from build123d import *

# Parameters (mm, degrees)
F0_W     = 180
F0_H     = 50
F1_DEPTH = 2.5
F3_DEPTH = 60
F5_DEPTH = 50
F6_W     = 7.071068
F6_H     = 5
F7_DEPTH = 25
F8_W     = 7.071068
F8_H     = 5
F9_DEPTH = 25


with BuildPart() as f1:
    # F0 (on Right) → F1 (new body, symmetric)
    with BuildSketch(Plane.YZ):
        Rectangle(F0_W, F0_H)
    extrude(amount=F1_DEPTH, both=True)

    # F2 (on face) → F3 (cut)
    with BuildSketch(Plane.XY.offset(25)):
        Polygon((-2.5, -85), (-2.5, -90), (2.5, -90), align=None)
    extrude(amount=-F3_DEPTH, mode=Mode.SUBTRACT)

    # F4 (on face) → F5 (cut)
    with BuildSketch(Plane.XY.offset(25)):
        Polygon((2.5, 90), (-2.5, 90), (-2.5, 85), align=None)
    extrude(amount=-F5_DEPTH, mode=Mode.SUBTRACT)

    # F6 (on face) → F7 (cut)
    with BuildSketch(Plane(origin=(-43.75, -43.75, 0), x_dir=(0.707107, -0.707107, 0), z_dir=(-0.707107, -0.707107, 0))):
        with Locations((61.871843, -2.5)):
            Rectangle(F6_W, F6_H)
        with Locations((61.871843, 2.5)):
            Rectangle(F6_W, F6_H)
    extrude(amount=-F7_DEPTH, mode=Mode.SUBTRACT)

    # F8 (on face) → F9 (cut)
    with BuildSketch(Plane(origin=(-43.75, 43.75, 0), x_dir=(-0.707107, -0.707107, 0), z_dir=(-0.707107, 0.707107, 0))):
        with Locations((-61.871843, -2.5)):
            Rectangle(F8_W, F8_H)
        with Locations((-61.871843, 2.5)):
            Rectangle(F8_W, F8_H)
    extrude(amount=-F9_DEPTH, mode=Mode.SUBTRACT)


solid = f1.part
The listing builds one solid part. Answer for the finished solid, in the listing's coordinates (mm). A direction names the side the tool comes from. Coordinates: 2 decimals unless noted, no trailing zeros. Order: outer loops, then holes, each group sorted by start corner. A loop starts at its lowest first (then second) coordinate and runs counter-clockwise, first axis right, second up.
Q1. Consider line 1 (Y direction, x = 0.95, z = -12); line 2 (Y direction, x = 1.25, z = -14.5). Determine where each line is inside the solid, lowest interval first.
Q2. A cutting plane is placed at B-B, the plane z = -16. Write down the section's boundary in (x, y), and give its area (3 significant figures).
Q3. Which of the six approach directions +Z, -Z, +X, -X, +Y, -Y give full straight-line access (tool end or side, diameter ignored) to faces 1 (the face through (1, -85, 5)), 2 (the face through (0, -1, -25)), 3 (the face through (1, 86, 5))?
Q4. A cutting plane is placed at A-A, the plane x = -0.2. Write down the section's boundary in (y, z), and give its area (3 significant figures).
Q5. Given P1, Ø1, axis at x = -0.5, z = -11, coming from the +Y side, flat-ended and moving along its own axis, determine where the tip first touches the part or whether it passes through.
Q6. For a pull along Z with two mould halves and no side action, classify faces 4 (the face through (0, 87.5, 15.1)), 5 (the face through (0, -1, 25)), 6 (the face through (0, -82.5, 0.1)), 7 (the face through (0, 82.5, -0.1)) as pulls with the +Z half, pulls with the -Z half, needs draft (parallel to the pull), parting line crosses it, or undercut.
Answers follow:
1. line 1: y = -88.45 to 88.45
1. line 2: y = -88.75 to 88.75
2. outline: (-2.5, -85) - (2.5, -90) - (2.5, 90) - (-2.5, 85) - close
2. area: 875 mm2
3. face 1: +X, -Y
3. face 2: -Z, +X, -X, +Y, -Y
3. face 3: +X, +Y
4. outline: (-87.3, -25) - (87.3, -25) - (87.3, -5) - (82.7, -5) - (82.7, 5) - (87.3, 5) - (87.3, 25) - (-87.3, 25) - (-87.3, 5) - (-82.7, 5) - (-82.7, -5) - (-87.3, -5) - close
4. area: 8,640 mm2
5. P1: stops at y = 87.5
6. face 4: needs draft
6. face 5: pulls with the +Z half
6. face 6: undercut
6. face 7: undercut
